Could you check a few things on this model? Use its own coordinates, in mm. Give positions to 0.01 mm unless a question says otherwise; leave off trailing zeros. Order: outer loops, then holes, each group sorted by start corner. A loop starts at its lowest first (then second) coordinate and runs counter-clockwise, first axis right, second up. Notation, with made-up numbers: (-1.75, 61.5) -> (56.25, 61.5) arc R21 ccw to (56.25, 84.5) -> close; hole circle Ø1 at (-2, 25). An arc over 180 degrees is marked (long way). Answer as CSV lines item,"result". Start each with the question number.
(1) I want a section at A-A (x = 0). Please give me the cut outline in (y, z), plus the area to 3 significant figures.
(2) Will these pins go through, and if not, where does the flat tip stop? pin 1 Ø3 at (x, z) = (2.5, -7) entering from -Y; pin 2 Ø6 at (y, z) = (-12, -29.5) entering from -X; pin 3 Ø10 at (x, z) = (-9.5, -103.5) entering from +Y.
(3) I want a section at C-C (z = 100). Please give me the cut outline in (x, y).
(4) I want a section at B-B (y = 0). Please give me the cut outline in (x, z).
(5) I need wall thicknesses on L1, parallel to Z at x = 0, y = -22; L2, parallel to Y at x = 0, z = 22; L3, parallel to X at y = -14, z = -88. Which ranges of each line are inside material? Lowest first, please.
(6) We'd pull the mould along Z, two halves only. Please class faces 1 (the face through (0.596, 22.369, -97.315)), 2 (the face through (-11, 17, 150)), 3 (the face through (23.846, 7.509, 2.1)): released by +Z, released by -Z, zero draft, split by the parting line, or undercut.
(7) I want a section at D-D (z = -37). Please give me the cut outline in (x, y), plus the area to 3 significant figures.
```python
from build123d import *

# Parameters (mm, degrees)
F0_R     = 25
F1_DEPTH = 150
F2_T     = -5
F5_D     = 5.5


with BuildPart() as f1:
    # F0 (on Top) → F1 (new body, symmetric)
    with BuildSketch(Plane.XY):
        Circle(F0_R)
    extrude(amount=F1_DEPTH, both=True)

    # F2
    f2_openings = [f1.faces().sort_by_distance(p)[0] for p in [
        (0, 0, 150),
        (0, 0, -150),
    ]]
    offset(amount=F2_T, openings=f2_openings)

    # F5 (through all)
    with Locations(Plane(origin=(0, 50, 0), x_dir=(1, 0, 0), z_dir=(0, 1, 0))):
        with Locations((0, 100), (0, -100)):
            Hole(F5_D / 2)


solid = f1.part
```
Final values:
1,outline,"(-25, -150) -> (-20, -150) -> (-20, -102.75) -> (-25, -102.75) -> close; (-25, -97.25) -> (-20, -97.25) -> (-20, 97.25) -> (-25, 97.25) -> close; (-25, 102.75) -> (-20, 102.75) -> (-20, 150) -> (-25, 150) -> close; (20, -150) -> (25, -150) -> (25, -102.75) -> (20, -102.75) -> close; (20, -97.25) -> (25, -97.25) -> (25, 97.25) -> (20, 97.25) -> close; (20, 102.75) -> (25, 102.75) -> (25, 150) -> (20, 150) -> close"
1,area,"2,890 mm²"
2,pin 1,"y = -24.98"
2,pin 2,"x = -23.32"
2,pin 3,"y = 24.59"
3,outline,"(-2.75, -24.85) -> (-2.75, -19.81) arc R20 cw to (-2.75, 19.81) -> (-2.75, 24.85) arc R25 ccw to start; (2.75, -24.85) arc R25 ccw to (2.75, 24.85) -> (2.75, 19.81) arc R20 cw to (2.75, -19.81) -> close"
4,outline,"(-25, -150) -> (-20, -150) -> (-20, 150) -> (-25, 150) -> close; (20, -150) -> (25, -150) -> (25, 150) -> (20, 150) -> close"
5,L1,"-150 to -102.75, -97.25 to 97.25, 102.75 to 150"
5,L2,"-25 to -20, 20 to 25"
5,L3,"-20.71 to -14.28, 14.28 to 20.71"
6,face 1,"undercut"
6,face 2,"released by +Z"
6,face 3,"zero draft"
7,outline,"circle Ø50 at (0, 0); hole circle Ø40 at (0, 0)"
7,area,"707 mm²"
